from build123d import *

# Parameters (mm, degrees)
CYLINDER001_R             = 0.7
CYLINDER001_DEPTH         = 2
CYLINDER001_ROLL_ANGLE    = 90
BOX005_W                  = 1
BOX005_H                  = 2
BOX005_DEPTH              = 3
FUSION002_PLACEMENT_ANGLE = 180
CYLINDER003_R             = 0.7
CYLINDER003_DEPTH         = 3
CYLINDER003_PITCH_ANGLE   = 90
BOX007_W                  = 3
BOX007_H                  = 1
BOX007_DEPTH              = 4.5
SKETCH023_W               = 1.2
SKETCH023_H               = 1.6
SKETCH023_W_2             = 1.6
SKETCH023_H_2             = 1.2
PAD005_DEPTH              = 1
FILLET010_R               = 0.3
PAD001_DEPTH              = 4
POCKET_DEPTH              = 1.5
POCKET001_DEPTH           = 3.5
SKETCH004_W               = 28
SKETCH004_H               = 42.5
POCKET002_DEPTH           = 0.7
POCKET005_DEPTH           = 1.5
FILLET007_R               = 0.3
PAD006_DEPTH              = 1
FILLET008_R               = 0.3
CYLINDER002_R             = 0.7
CYLINDER002_DEPTH         = 2
CYLINDER002_ROLL_ANGLE    = 90
BOX006_W                  = 1
BOX006_H                  = 2
BOX006_DEPTH              = 3


with BuildPart() as cylinder:
    # Cylinder001 → Cylinder001 (new body)
    with BuildSketch(Plane.XY):
        Circle(CYLINDER001_R)
    extrude(amount=CYLINDER001_DEPTH)


with BuildPart() as cylinder_1:
    # Cylinder001 roll: moved
    add(cylinder.part.rotate(Axis((0, 0, 0), (1, 0, 0)), CYLINDER001_ROLL_ANGLE))


with BuildPart() as cylinder_2:
    # Cylinder001 placement: moved
    add(cylinder_1.part.moved(Location((-0.2, 42, 1.8))))


with BuildPart() as fusion002:
    # Box005 → Box005 (new body)
    with BuildSketch(Plane(origin=(-0.1, 40, -1), x_dir=(1, 0, 0), z_dir=(0, 0, 1))):
        with Locations((0.5, 1)):
            Rectangle(BOX005_W, BOX005_H)
    extrude(amount=BOX005_DEPTH)

    # Fusion002: union Cylinder
    add(cylinder_2.part)


with BuildPart() as fusion002_1:
    # Fusion002 placement: moved
    add(fusion002.part.moved(Location((27.5, 82, 0))).rotate(Axis((27.5, 82, 0), (0, 0, 1)), FUSION002_PLACEMENT_ANGLE))


with BuildPart() as cylinder002:
    # Cylinder003 → Cylinder003 (new body)
    with BuildSketch(Plane.XY):
        Circle(CYLINDER003_R)
    extrude(amount=CYLINDER003_DEPTH)


with BuildPart() as cylinder002_1:
    # Cylinder003 pitch: moved
    add(cylinder002.part.rotate(Axis((0, 0, 0), (0, 1, 0)), CYLINDER003_PITCH_ANGLE))


with BuildPart() as cylinder002_2:
    # Cylinder003 placement: moved
    add(cylinder002_1.part.moved(Location((12.25, -1.9, 1.85))))


with BuildPart() as fusion_conn_top:
    # Box007 → Box007 (new body)
    with BuildSketch(Plane(origin=(12.25, -1.7, -2), x_dir=(1, 0, 0), z_dir=(0, 0, 1))):
        with Locations((1.5, 0.5)):
            Rectangle(BOX007_W, BOX007_H)
    extrude(amount=BOX007_DEPTH)

    # Fusion004: union Cylinder002
    add(cylinder002_2.part)


with BuildPart() as fillet010:
    # Sketch023 → Pad005 (new body)
    with BuildSketch(Plane.XY):
        with Locations((4.2, -0.45)):
            Rectangle(SKETCH023_W, SKETCH023_H)
        with Locations((23.2, -0.45)):
            Rectangle(SKETCH023_W, SKETCH023_H)
        with Locations((-0.45, 37.4)):
            Rectangle(SKETCH023_W_2, SKETCH023_H_2)
        with Locations((27.95, 37.4)):
            Rectangle(SKETCH023_W_2, SKETCH023_H_2)
    extrude(amount=PAD005_DEPTH)

    # Fillet010
    fillet010_edges = [fillet010.edges().sort_by_distance(p)[0] for p in [
        (27.15, 37.4, 0),
        (27.15, 37.4, 1),
        (0.35, 37.4, 0),
        (0.35, 37.4, 1),
        (4.2, 0.35, 0),
        (4.2, 0.35, 1),
        (23.2, 0.35, 0),
        (23.2, 0.35, 1),
    ]]
    fillet(fillet010_edges, radius=FILLET010_R)


with BuildPart() as fillet007_top:
    # Sketch → Pad001 (new body)
    with BuildSketch(Plane(origin=(13.75, 21, -4), x_dir=(1, 0, 0), z_dir=(0, 0, 1))):
        with BuildLine():
            ThreePointArc((16, 22), (0, 24.8188), (-16, 22))
            Line((-16, 22), (-16, -22))
            ThreePointArc((-16, -22), (0, -24.8188), (16, -22))
            Line((16, -22), (16, 22))
        make_face()
    extrude(amount=PAD001_DEPTH)

    # Sketch002 → Pocket (cut)
    with BuildSketch(Plane(origin=(13.75, 21, -4), x_dir=(1, 0, 0), z_dir=(0, 0, -1))):
        with BuildLine():
            Line((-13.5, 21), (13.5, 21))
            ThreePointArc((14, 20.5), (13.853553, 20.853553), (13.5, 21))
            Line((14, 20.5), (14, -20.5))
            ThreePointArc((13.5, -21), (13.853553, -20.853553), (14, -20.5))
            Line((13.5, -21), (-13.5, -21))
            ThreePointArc((-14, -20.5), (-13.853553, -20.853553), (-13.5, -21))
            Line((-14, -20.5), (-14, 20.5))
            ThreePointArc((-13.5, 21), (-13.853553, 20.853553), (-14, 20.5))
        make_face()
    extrude(amount=-POCKET_DEPTH, mode=Mode.SUBTRACT)

    # Sketch003 → Pocket001 (cut)
    with BuildSketch(Plane(origin=(13.75, 21, 0), x_dir=(1, 0, 0), z_dir=(0, 0, 1))):
        Polygon((-13.5, -19), (-13.5, 11.5), (-12.5, 11.5), (-12.5, 20), (12.5, 20), (12.5, 11.5), (13.5, 11.5), (13.5, -19), (12.5, -19), (12.5, -20), (-12.5, -20), (-12.5, -19), align=None)
    extrude(amount=-POCKET001_DEPTH, mode=Mode.SUBTRACT)

    # Sketch004 → Pocket002 (cut)
    with BuildSketch(Plane(origin=(13.75, 21, 0), x_dir=(1, 0, 0), z_dir=(0, 0, 1))):
        Rectangle(SKETCH004_W, SKETCH004_H)
    extrude(amount=-POCKET002_DEPTH, mode=Mode.SUBTRACT)

    # Sketch008 → Pocket005 (cut)
    with BuildSketch(Plane(origin=(13.75, 21, 0), x_dir=(1, 0, 0), z_dir=(0, 0, 1))):
        with BuildLine():
            ThreePointArc((12, 19.621417), (0, 23), (-12, 19.621417))
            Line((-12, 19.621417), (12, 19.621417))
        make_face()
        with BuildLine():
            ThreePointArc((-12, -19.621417), (0, -23), (12, -19.621417))
            Line((-12, -19.621417), (12, -19.621417))
        make_face()
    extrude(amount=-POCKET005_DEPTH, mode=Mode.SUBTRACT)

    # Fillet007
    fillet007_edges = [fillet007_top.edges().sort_by_distance(p)[0] for p in [
        (-2.25, 21, -4),
        (-2.25, 43, -2),
        (13.75, 45.8188, -4),
        (29.75, 43, -2),
        (29.75, 21, -4),
        (29.75, -1, -2),
        (13.75, -3.8188, -4),
        (-2.25, -1, -2),
    ]]
    fillet(fillet007_edges, radius=FILLET007_R)


with BuildPart() as fillet008_hanger_top:
    # Sketch019 → Pad006 (new body)
    with BuildSketch(Plane(origin=(13.5, 1, -1), x_dir=(1, 0, 0), z_dir=(0, 0, 1))):
        with BuildLine():
            ThreePointArc((5, 48), (0, 48.266714), (-5, 48))
            Line((-5, 48), (-5, 44))
            Line((-5, 44), (-3.5, 44))
            Line((-3.5, 47), (-3.5, 44))
            ThreePointArc((3.5, 47), (0, 47.130139), (-3.5, 47))
            Line((3.5, 44), (3.5, 47))
            Line((5, 44), (3.5, 44))
            Line((5, 48), (5, 44))
        make_face()
    extrude(amount=PAD006_DEPTH)

    # Fillet008
    fillet008_edges = [fillet008_hanger_top.edges().sort_by_distance(p)[0] for p in [
        (18.5, 47, -1),
        (17, 46.5, -1),
        (18.5, 49, -0.5),
        (13.5, 49.266714, -1),
        (13.5, 48.130139, -1),
        (10, 46.5, -1),
        (8.5, 47, -1),
        (8.5, 49, -0.5),
    ]]
    fillet(fillet008_edges, radius=FILLET008_R)


with BuildPart() as cylinder001:
    # Cylinder002 → Cylinder002 (new body)
    with BuildSketch(Plane.XY):
        Circle(CYLINDER002_R)
    extrude(amount=CYLINDER002_DEPTH)


with BuildPart() as cylinder001_1:
    # Cylinder002 roll: moved
    add(cylinder001.part.rotate(Axis((0, 0, 0), (1, 0, 0)), CYLINDER002_ROLL_ANGLE))


with BuildPart() as cylinder001_2:
    # Cylinder002 placement: moved
    add(cylinder001_1.part.moved(Location((-0.2, 42, 1.8))))


with BuildPart() as fusion016:
    # Box006 → Box006 (new body)
    with BuildSketch(Plane(origin=(-0.1, 40, -1), x_dir=(1, 0, 0), z_dir=(0, 0, 1))):
        with Locations((0.5, 1)):
            Rectangle(BOX006_W, BOX006_H)
    extrude(amount=BOX006_DEPTH)

    # Fusion015: union Cylinder001
    add(cylinder001_2.part)

    # Fusion016: union Fusion002, Fusion-conn-top, Fillet010, Fillet007-top, Fillet008-hanger-top
    add(fusion002_1.part)
    add(fusion_conn_top.part)
    add(fillet010.part)
    add(fillet007_top.part)
    add(fillet008_hanger_top.part)


with BuildPart() as fusion016_1:
    # Fusion016 placement: moved
    add(fusion016.part.moved(Location((0, 0, -4))))


solid = fusion016_1.part
Geometry: final body of the model. Coordinates: model frame, mm. A direction names the side the tool comes from. Round coordinates to 2 decimals unless told otherwise and drop trailing zeros. Write each loop counter-clockwise with the first axis right and the second up, starting at its lowest first coordinate (ties: lowest second). Pieces come first, ordered by that corner, then holes. Notation, with made-up numbers: M -38.5,86 L -9.5,86 A21 ccw -9.5,103 Z; hole C 9,2.5 d5. An arc over 180 degrees is marked long. Write item = value, one per line.
Item 1: Material intervals for line 1 along X through (y, z) = (40.5, -5); line 2 along X through (y, z) = (24, -4.5); line 3 along Z through (x, y) = (-0.5, 36.5), sorted ascending. Write a range as [from, to].
Findings:
line_1 = [-2.25, 1.25], [26.25, 29.75]
line_2 = [-2.25, -0.25], [27.75, 29.75]
line_3 = [-8, -4]
Item 2: Section query B-B on z = -7. Return loops of the section in (x, y), then the cut area to 3 significant figures.
Findings:
outline = M -2.25,-0.79 A0.3 ccw -2.05,-1.07 A46.82 ccw 29.55,-1.07 A0.3 ccw 29.75,-0.79 L 29.75,42.79 A0.3 ccw 29.55,43.07 A46.82 ccw -2.05,43.07 A0.3 ccw -2.25,42.79 Z; hole M -0.25,0.5 A0.5 ccw 0.25,0 L 27.25,0 A0.5 ccw 27.75,0.5 L 27.75,41.5 A0.5 ccw 27.25,42 L 0.25,42 A0.5 ccw -0.25,41.5 Z
area = 353 mm^2
Item 3: Section query A-A on y = 33.5. Return loops of the section in (x, z), then the cut area to 3 significant figures.
Findings:
outline = M -2.25,-7.7 A0.3 ccw -1.95,-8 L -0.25,-8 L -0.25,-6.5 L 1.25,-6.5 L 1.25,-4.7 L -0.25,-4.7 L -0.25,-4 L -2.25,-4 Z; M 26.25,-6.5 L 27.75,-6.5 L 27.75,-8 L 29.45,-8 A0.3 ccw 29.75,-7.7 L 29.75,-4 L 27.75,-4 L 27.75,-4.7 L 26.25,-4.7 Z
area = 21.4 mm^2
Item 4: Pull-direction query (Y, two-part tool) for faces 1 (the face through (27, 40, -3)), 2 (the face through (22.6, -0.5, -3.5)), 3 (the face through (23.2, -1.25, -3.5)); classes: pulls with the +Y half, pulls with the -Y half, needs draft (parallel to the pull), parting line crosses it, or undercut.
Findings:
face_1 = undercut
face_2 = needs draft
face_3 = pulls with the -Y half
Item 5: Pin query (flat end, axial travel): P1, Ø2.5, axis at x = 11.5, y = 0, coming from the +Z side; P2, Ø2, axis at x = 17.5, y = 42, coming from the +Z side; P3, Ø3, axis at x = 2, z = -4, coming from the -Y side. Return the tip coordinate at first contact, or that it passes through.
Findings:
P1 = -1.5
P2 = -5.5
P3 = -2.68
Item 6: Section query C-C on y = 14.5. Return loops of the section in (x, z), then the cut area to 3 significant figures.
Findings:
outline = M -2.25,-7.7 A0.3 ccw -1.95,-8 L -0.25,-8 L -0.25,-6.5 L 0.25,-6.5 L 0.25,-4.7 L -0.25,-4.7 L -0.25,-4 L -2.25,-4 Z; M 27.25,-6.5 L 27.75,-6.5 L 27.75,-8 L 29.45,-8 A0.3 ccw 29.75,-7.7 L 29.75,-4 L 27.75,-4 L 27.75,-4.7 L 27.25,-4.7 Z
area = 17.8 mm^2
Item 7: Access query for faces 4 (the face through (4.8, -0.5, -3.5)), 5 (the face through (14, -1, -1.5)), 6 (the face through (4, -1, -3)). Directions: +Z, -Z, +X, -X, +Y, -Y. A direction counts if a zero-diameter tool reaches every point of the face in a straight line with its end or side. Return the directions, or none.
Findings:
face_4 = +Z, +Y, -Y
face_5 = +Z, +X, -X, +Y
face_6 = +Z, -X, +Y, -Y
